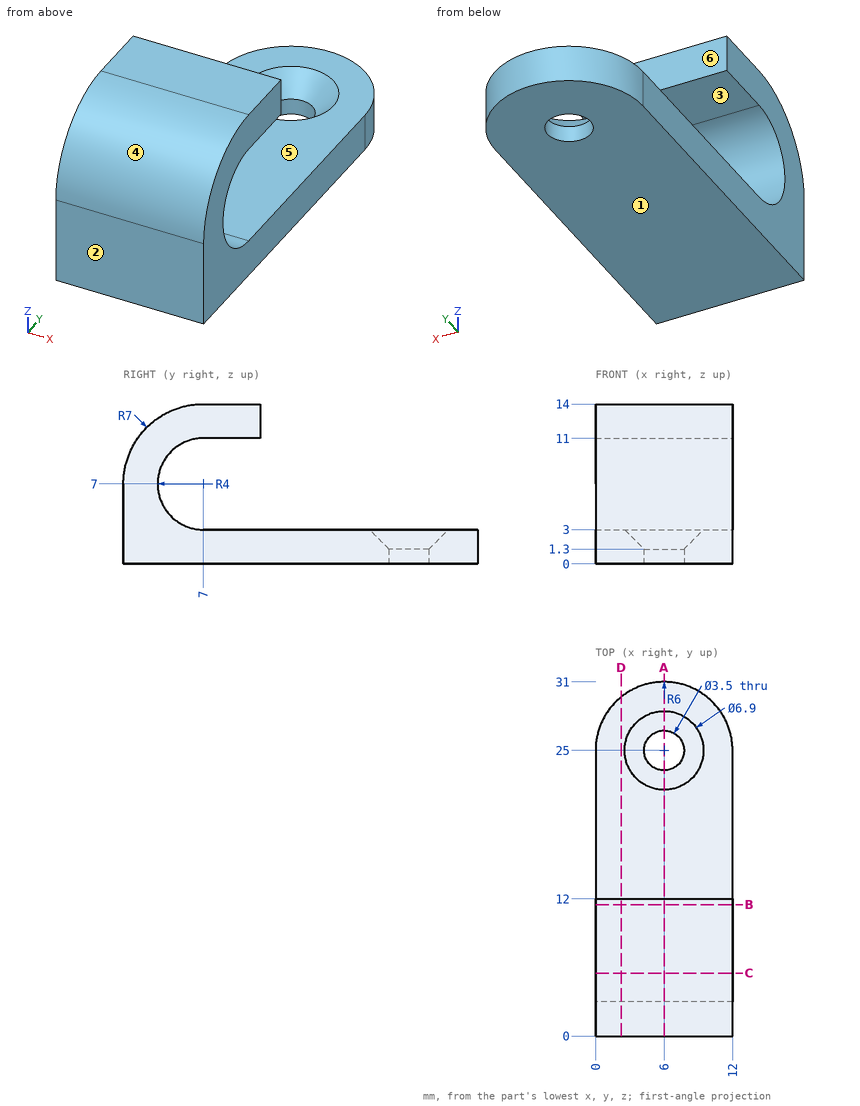
Drawing for the job (mm, zero at the part's lowest x, y, z). A direction names the side the tool comes from. Round coordinates to 2 decimals unless told otherwise and drop trailing zeros. Loops run counter-clockwise (first coordinate to the right, second up) from the corner with the lowest first, then second, coordinate; pieces in that order, holes last. Notation, with made-up numbers: (3, -34) - (47, -34) arc R23 cw to (47, -8) - close; hole circle Ø11 at (-22.5, 47.25). An arc over 180 degrees is marked (long way). Return JSON: item names as keys, results as strings. Group by question number.
Q1. Band-saw the part on D-D on x = 2.25. Give the cut face in (y, z), plus the area to 3 significant figures.
Q2. Band-saw the part on C-C on y = 5.5. Give the cut face in (x, z), plus the area to 3 significant figures.
Q3. Drill centre lines: line 1 along Z through (x, y) = (7, 9.5); line 2 along Y through (x, z) = (6, 0.9); line 3 along Z through (x, y) = (1.5, 16.5). Where is each one in solid material? Low to high. Write a range as [from, to].
Q4. Band-saw the part on B-B on y = 11.5. Give the cut face in (x, z), plus the area to 3 significant figures.
Q5. Flat gauge pins, fed straight in: pin 1 Ø1.5 at (x, y) = (10.5, 4) entering from +Z; pin 2 Ø1.5 at (x, y) = (8.5, 9) entering from -Z; pin 3 Ø1 at (x, z) = (5, 4.5) entering from +Y; pin 4 Ø3.5 at (x, y) = (3, 19) entering from +Z. Where does each tip first touch, or does it go through?
Q6. Two-plate mould, pull along Z, no slides. Class the marked faces 1, 2 and 3: +Z half, -Z half, draft (parallel to the pull), parting line (faces both ways), or undercut.
Q7. Tool access for the marked faces 4, 5 and 6: list every direction of +Z, -Z, +X, -X, +Y, -Y with a clear straight run to the whole face (end or side of a thin tool).
Q8. Band-saw the part on A-A on x = 6. Give the cut face in (y, z).
Solutions:
{
 "1": {"outline": "(0, 0) - (29.68, 0) - (29.68, 3) - (7, 3) arc R4 cw to (7, 11) - (12, 11) - (12, 14) - (7, 14) arc R7 ccw to (0, 7) - close", "area": "145 mm^2"},
 "2": {"outline": "(0, 0) - (12, 0) - (12, 3.29) - (0, 3.29) - close; (0, 10.71) - (12, 10.71) - (12, 13.84) - (0, 13.84) - close", "area": "77.1 mm^2"},
 "3": {"line 1": "z = [0, 3], [11, 14]", "line 2": "y = [0, 23.25], [26.75, 31]", "line 3": "z = [0, 3]"},
 "4": {"outline": "(0, 0) - (12, 0) - (12, 3) - (0, 3) - close; (0, 11) - (12, 11) - (12, 14) - (0, 14) - close", "area": "72.0 mm^2"},
 "5": {"pin 1": "stops at z = 13.63", "pin 2": "stops at z = 0", "pin 3": "stops at y = 4.35", "pin 4": "stops at z = 3"},
 "6": {"face 1": "-Z half", "face 2": "draft", "face 3": "undercut"},
 "7": {"face 4": "+Z, +X, -X, -Y", "face 5": "+X, -X, +Y", "face 6": "+Z, +X, -X, +Y"},
 "8": {"outline": "(0, 0) - (23.25, 0) - (23.25, 1.3) - (21.55, 3) - (7, 3) arc R4 cw to (7, 11) - (12, 11) - (12, 14) - (7, 14) arc R7 ccw to (0, 7) - close; (26.75, 0) - (31, 0) - (31, 3) - (28.45, 3) - (26.75, 1.3) - close"}
}
